```python
from build123d import *

# Parameters (mm, degrees)
CYLINDER045_R          = 1.38
CYLINDER045_DEPTH      = 10
CYLINDER044_R          = 1.38
CYLINDER044_DEPTH      = 10
BOX026_W               = 25
BOX026_H               = 10
BOX026_DEPTH           = 4
CUT024_PLACEMENT_ANGLE = 30
FILLET001_R            = 3


with BuildPart() as cylinder045:
    # Cylinder045 → Cylinder045 (new body)
    with BuildSketch(Plane(origin=(25, 52, 59), x_dir=(1, 0, 0), z_dir=(0, 0, 1))):
        Circle(CYLINDER045_R)
    extrude(amount=CYLINDER045_DEPTH)


with BuildPart() as cylinder044:
    # Cylinder044 → Cylinder044 (new body)
    with BuildSketch(Plane(origin=(40, 52, 59), x_dir=(1, 0, 0), z_dir=(0, 0, 1))):
        Circle(CYLINDER044_R)
    extrude(amount=CYLINDER044_DEPTH)


with BuildPart() as fillet001:
    # Box026 → Box026 (new body)
    with BuildSketch(Plane(origin=(45, 57, 62), x_dir=(-1, 0, 0), z_dir=(0, 0, 1))):
        with Locations((12.5, 5)):
            Rectangle(BOX026_W, BOX026_H)
    extrude(amount=BOX026_DEPTH)

    # Cut025: cut Cylinder044
    add(cylinder044.part, mode=Mode.SUBTRACT)

    # Cut024: cut Cylinder045
    add(cylinder045.part, mode=Mode.SUBTRACT)


with BuildPart() as fillet001_1:
    # Cut024 placement: moved
    add(fillet001.part.moved(Location((-20.65, 26.95, 0))).rotate(Axis((-20.65, 26.95, 0), (0, 0, -1)), CUT024_PLACEMENT_ANGLE))

    # Fillet001
    fillet001_edges = [fillet001_1.edges().sort_by_distance(p)[0] for p in [
        (25.170508, 66.313448, 64),
        (20.170508, 57.653194, 64),
    ]]
    fillet(fillet001_edges, radius=FILLET001_R)


with BuildPart() as fillet001_2:
    # Fillet001 placement: moved
    add(fillet001_1.part.moved(Location((-2, 5, 0))))


solid = fillet001_2.part
```
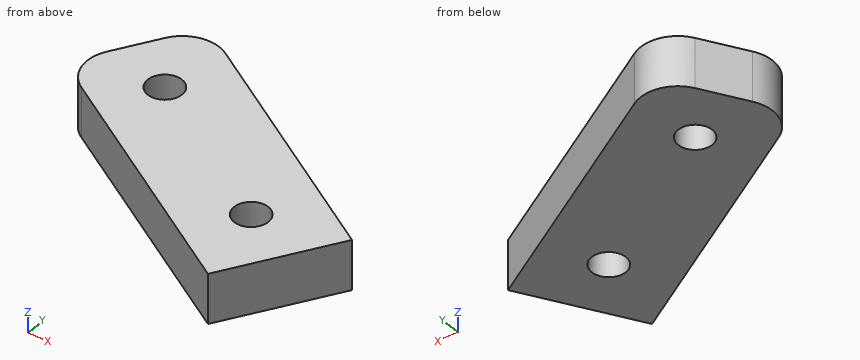
The listing builds one solid part. Answer for the finished solid, in the listing's coordinates (mm). Coordinates: 2 decimals unless noted, no trailing zeros. Write each loop counter-clockwise with the first axis right and the second up, starting at its lowest first coordinate (ties: lowest second). Pieces come first, ordered by that corner, then holes. Notation, with made-up numbers: (2.5, 23.25) - (29.5, 23.25) arc R33 cw to (29.5, 52.25) - close; hole circle Ø4 at (18.25, 84). An arc over 180 degrees is marked (long way). Return JSON: item names as keys, results as strings. Group by question number.
1. A cutting plane is placed at C-C, the plane y = 56.75. Determine the outline of the cut face in (x, z).
2. A cutting plane is placed at D-D, the plane y = 54. Determine the outline of the cut face in (x, z), plus the area to 3 significant figures.
3. A cutting plane is placed at B-B, the plane z = 62.8. Determine the outline of the cut face in (x, y), plus the area to 3 significant figures.
4. Straight lines are drawn through the part: L1, parallel to X at y = 56.5, z = 64.6; L2, parallel to X at y = 63.5, z = 65.2; L3, parallel to Y at x = 27.25, z = 63.6. For each, find the intervals that lie inside material, in ascending order.
5. Given pin 1 (1 mm diameter, centred on x = 32, z = 64.5, fed in from -Y); pin 2 (2 mm diameter, centred on x = 26, y = 56.5, fed in from +Z), each flat-ended and moving along its own axis, determine where each tip first touches the part or whether it passes through.
6. A cutting plane is placed at A-A, the plane x = 37. Determine the outline of the cut face in (y, z), plus the area to 3 significant figures.
Ans:
{
 "1": {"outline": "(28.4, 62) - (36.63, 62) - (36.63, 66) - (28.4, 66) - close; (39.35, 62) - (43.63, 62) - (43.63, 66) - (39.35, 66) - close"},
 "2": {"outline": "(33.16, 62) - (42.04, 62) - (42.04, 66) - (33.16, 66) - close", "area": "35.5 mm²"},
 "3": {"outline": "(19.67, 65.25) arc R3 ccw to (20.77, 61.15) - (39.82, 50.15) - (44.82, 58.81) - (25.77, 69.81) arc R3 ccw to (21.67, 68.72) - close; hole circle Ø2.76 at (25, 64.48); hole circle Ø2.76 at (37.99, 56.98)", "area": "234 mm²"},
 "4": {"L1": "28.83 to 36.7, 39.28 to 43.49", "L2": "19.28 to 24.03, 25.97 to 36.7", "L3": "57.41 to 68.96"},
 "5": {"pin 1": "y = 54.38", "pin 2": "through"},
 "6": {"outline": "(51.78, 62) - (56.02, 62) - (56.02, 66) - (51.78, 66) - close; (57.94, 62) - (63.33, 62) - (63.33, 66) - (57.94, 66) - close", "area": "38.5 mm²"}
}
